Read the model definition and answer for the solid it produces. Units are mm, in the model's axes. A direction names the side the tool comes from. Coordinates: 2 decimals unless noted, no trailing zeros. Loops run counter-clockwise (first coordinate to the right, second up) from the corner with the lowest first, then second, coordinate; pieces in that order, holes last. Notation, with made-up numbers: (-3, -7) -> (23, -7) arc R14 cw to (23, -2) -> close; hole circle Ø11 at (-7.75, 87.5). An arc over 180 degrees is marked (long way). Answer in a Markdown table with one row per item.
```python
from build123d import *

# Parameters (mm, degrees)
SKETCH2_W           = 25
SKETCH2_H           = 25
SKETCH2_W_2         = 21
SKETCH2_H_2         = 21
EXTRUDE_THIN1_DEPTH = 125
SKETCH3_R           = 4
HOLE_DEPTH          = 129.086884574


with BuildPart() as part:
    # Sketch2 → Extrude-Thin1 (new, symmetric)
    with BuildSketch(Plane.XY):
        Rectangle(SKETCH2_W, SKETCH2_H)
        Rectangle(SKETCH2_W_2, SKETCH2_H_2, mode=Mode.SUBTRACT)
    extrude(amount=EXTRUDE_THIN1_DEPTH, both=True)

    # Sketch3 → hole (cut, through all)
    with BuildSketch(Plane(origin=(12.5, 0, 0), x_dir=(0, 0, -1), z_dir=(1, 0, 0))):
        with Locations((105, 0)):
            Circle(SKETCH3_R)
    extrude(amount=-HOLE_DEPTH, mode=Mode.SUBTRACT)


solid = part.part
```
1. A tool of negligible diameter and unlimited length cuts with its end or side. For faces 5 (the flat face through (-10.5, 0, 2)), 6 (the flat face through (0, -12.5, 2)), from which of +Z, -Z, +X, -X, +Y, -Y can it reach the whole face along a straight path? Write none if from no direction.
A:
| item | result |
|---|---|
| face 5 | +Z, -Z |
| face 6 | +Z, -Z, +X, -X, -Y |
2. The mould has two halves that part along X. Classify faces 1 (the flat face through (-12.5, 0, 2)), 2 (the flat face through (0, 12.5, 2)), 3 (the flat face through (10.5, 0, 2)), 4 (the flat face through (0, 10.5, 2)): pulls with the +X half, pulls with the -X half, needs draft (parallel to the pull), parting line crosses it, or undercut.
A:
| item | result |
|---|---|
| face 1 | pulls with the -X half |
| face 2 | needs draft |
| face 3 | undercut |
| face 4 | undercut |
3. A cutting plane is placed at D-D on z = -38. Give the vertices of the cut face in (x, y).
A:
| item | result |
|---|---|
| outline | (-12.5, -12.5) -> (12.5, -12.5) -> (12.5, 12.5) -> (-12.5, 12.5) -> close; hole (-10.5, -10.5) -> (10.5, -10.5) -> (10.5, 10.5) -> (-10.5, 10.5) -> close |
4. A cutting plane is placed at A-A on y = -6.5. Give the vertices of the cut face in (x, z).
A:
| item | result |
|---|---|
| outline | (-12.5, -125) -> (-10.5, -125) -> (-10.5, 125) -> (-12.5, 125) -> close; (10.5, -125) -> (12.5, -125) -> (12.5, 125) -> (10.5, 125) -> close |
5. Find the intervals of material crossed by probe 1 along X at (y, z) = (3, 3.5); probe 2 along Y at (x, z) = (10.9, -105), in increasing order.
A:
| item | result |
|---|---|
| probe 1 | x = -12.5 to -10.5, 10.5 to 12.5 |
| probe 2 | y = -12.5 to -4, 4 to 12.5 |
6. A cutting plane is placed at B-B on z = -105. Give the vertices of the cut face in (x, y).
A:
| item | result |
|---|---|
| outline | (-12.5, -12.5) -> (12.5, -12.5) -> (12.5, -4) -> (10.5, -4) -> (10.5, -10.5) -> (-10.5, -10.5) -> (-10.5, -4) -> (-12.5, -4) -> close; (-12.5, 4) -> (-10.5, 4) -> (-10.5, 10.5) -> (10.5, 10.5) -> (10.5, 4) -> (12.5, 4) -> (12.5, 12.5) -> (-12.5, 12.5) -> close |
